from build123d import *

# Parameters (mm, degrees)
BOSS_EXTRUDE1_DEPTH       = 3
BOSS_EXTRUDE1_DEPTH_BACK  = 3
SKETCH2_R                 = 4.5
BOSS_EXTRUDE4_START       = -8.5
SKETCH2_6_R               = 6.5
SKETCH2_6_R_2             = 4.5
BOSS_EXTRUDE4_DEPTH       = 17
BOSS_EXTRUDE2_DEPTH       = 8.5
BOSS_EXTRUDE2_DEPTH_BACK  = 8.5
M2_TAPPED_HOLE1_REACH     = 63.876
M2_TAPPED_HOLE1_BORE_R    = 1.25
M2_TAPPED_HOLE2_REACH     = 59.753
M2_TAPPED_HOLE2_BORE_R    = 1.25
M3X0_5_TAPPED_HOLE1_D     = 2.5
M3X0_5_TAPPED_HOLE1_DEPTH = 7.5
M3X0_5_TAPPED_HOLE1_TIP   = 0.751075774
M3X0_5_TAPPED_HOLE2_D     = 2.5
M3X0_5_TAPPED_HOLE2_DEPTH = 7.5
M3X0_5_TAPPED_HOLE2_TIP   = 0.751075774


with BuildPart() as part:
    # Sketch2 → Boss-Extrude1 (new, two sides: drawn at the far end of the back side and taken through both)
    with BuildSketch(Plane(origin=(0, 0, 0), x_dir=(0, 0, -1), z_dir=(1, 0, 0)).offset(-BOSS_EXTRUDE1_DEPTH_BACK)):
        with BuildLine():
            ThreePointArc((0.33951151, -17.055452752), (1.492864746, -16.361954251), (1.94565571, -15.094616806))
            Line((1.94565571, -15.094616806), (1.94565571, -12.094616806))
            ThreePointArc((1.94565571, -12.094616806), (2.040471682, -11.22885835), (2.320424562, -10.404143759))
            Line((2.320424562, -10.404143759), (11.713700119, 9.73980068))
            ThreePointArc((11.713700119, 9.73980068), (12.140663851, 10.020732686), (12.599964806, 10.244927809))
            ThreePointArc((12.599964806, 10.244927809), (13.500806616, 10.98137419), (13.839273926, 12.094616806))
            Line((13.839273926, 12.094616806), (13.839273926, 15.094616806))
            ThreePointArc((13.839273926, 15.094616806), (13.500806616, 16.207859421), (12.599964806, 16.944305803))
            ThreePointArc((12.599964806, 16.944305803), (11.821767305, 17.370774506), (11.156747464, 17.958324943))
            ThreePointArc((11.156747464, 17.958324943), (9.9384514, 19.007187499), (8.5, 19.724972654))
            Line((8.5, 19.724972654), (8.5, 51.177740757))
            ThreePointArc((8.5, 51.177740757), (7.328427125, 54.006167882), (4.5, 55.177740757))
            Line((4.5, 55.177740757), (-4.5, 55.177740757))
            ThreePointArc((-4.5, 55.177740757), (-7.328427125, 54.006167882), (-8.5, 51.177740757))
            Line((-8.5, 51.177740757), (-8.5, -2.847998534))
            Line((-8.5, -2.847998534), (-12.230274542, -10.847598104))
            ThreePointArc((-12.230274542, -10.847598104), (-10.052447802, -18.929627561), (-1.717156713, -18.164740706))
            ThreePointArc((-1.717156713, -18.164740706), (-0.771632326, -17.45656389), (0.33951151, -17.055452752))
        make_face()
        with Locations((-6.339273926, -13.594616806)):
            Circle(SKETCH2_R, mode=Mode.SUBTRACT)
        with Locations((6.339273926, 13.594616806)):
            Circle(SKETCH2_R, mode=Mode.SUBTRACT)
    extrude(amount=BOSS_EXTRUDE1_DEPTH + BOSS_EXTRUDE1_DEPTH_BACK)

    # Sketch2<6> → Boss-Extrude4 (add)
    # profile 1 of 2: a face of its own
    with BuildSketch(Plane(origin=(0, 0, 0), x_dir=(0, 0, -1), z_dir=(1, 0, 0)).offset(BOSS_EXTRUDE4_START)):
        with BuildLine():
            ThreePointArc((11.156747464, 9.230908668), (11.423199363, 9.498514711), (11.713700119, 9.73980068))
            ThreePointArc((11.713700119, 9.73980068), (12.140663851, 10.020732686), (12.599964806, 10.244927809))
            ThreePointArc((12.599964806, 10.244927809), (13.500806616, 10.98137419), (13.839273926, 12.094616806))
            Line((13.839273926, 12.094616806), (13.839273926, 15.094616806))
            ThreePointArc((13.839273926, 15.094616806), (13.500806616, 16.207859421), (12.599964806, 16.944305803))
            ThreePointArc((12.599964806, 16.944305803), (11.821767305, 17.370774506), (11.156747464, 17.958324943))
            ThreePointArc((11.156747464, 17.958324943), (12.404073098, 15.933037427), (12.839273926, 13.594616806))
            ThreePointArc((12.839273926, 13.594616806), (12.404073098, 11.256196185), (11.156747464, 9.230908668))
        make_face()
    # profile 2 of 2: a face of its own
    with BuildSketch(Plane(origin=(0, 0, 0), x_dir=(0, 0, -1), z_dir=(1, 0, 0)).offset(BOSS_EXTRUDE4_START)):
        with Locations((6.339273926, 13.594616806)):
            Circle(SKETCH2_6_R)
        with Locations((6.339273926, 13.594616806)):
            Circle(SKETCH2_6_R_2, mode=Mode.SUBTRACT)
    extrude(amount=BOSS_EXTRUDE4_DEPTH)

    # Sketch2<4> → Boss-Extrude2 (add, two sides: drawn at the far end of the back side and taken through both)
    with BuildSketch(Plane(origin=(0, 0, 0), x_dir=(0, 0, -1), z_dir=(1, 0, 0)).offset(-BOSS_EXTRUDE2_DEPTH_BACK)):
        with BuildLine():
            Line((-8.5, 51.177740757), (-8.5, 30.594616806))
            ThreePointArc((-8.5, 30.594616806), (-7.328427125, 27.766189681), (-4.5, 26.594616806))
            Line((-4.5, 26.594616806), (4.5, 26.594616806))
            ThreePointArc((4.5, 26.594616806), (7.328427125, 27.766189681), (8.5, 30.594616806))
            Line((8.5, 30.594616806), (8.5, 51.177740757))
            ThreePointArc((8.5, 51.177740757), (7.328427125, 54.006167882), (4.5, 55.177740757))
            Line((4.5, 55.177740757), (-4.5, 55.177740757))
            ThreePointArc((-4.5, 55.177740757), (-7.328427125, 54.006167882), (-8.5, 51.177740757))
        make_face()
    extrude(amount=BOSS_EXTRUDE2_DEPTH + BOSS_EXTRUDE2_DEPTH_BACK)

    # M2 Tapped Hole1 bore → M2 Tapped Hole1 (cut, up to next)
    with BuildSketch(Plane(origin=(0, 0, -13.839273926), x_dir=(-1, 0, 0), z_dir=(0, 0, -1)), mode=Mode.PRIVATE) as m2_tapped_hole1_sk1:
        with Locations((0, 13.594616806)):
            Circle(M2_TAPPED_HOLE1_BORE_R)
    m2_tapped_hole1_tool1 = extrude(m2_tapped_hole1_sk1.sketch, amount=-M2_TAPPED_HOLE1_REACH, mode=Mode.PRIVATE) & part.part
    add(m2_tapped_hole1_tool1.solids().sort_by_distance((0, 13.594617, -13.839274))[0], mode=Mode.SUBTRACT)

    # M2 Tapped Hole2 bore → M2 Tapped Hole2 (cut, up to next)
    with BuildSketch(Plane(origin=(0, 0, -1.94565571), x_dir=(-1, 0, 0), z_dir=(0, 0, -1)), mode=Mode.PRIVATE) as m2_tapped_hole2_sk1:
        with Locations((0, -13.594616806)):
            Circle(M2_TAPPED_HOLE2_BORE_R)
    m2_tapped_hole2_tool1 = extrude(m2_tapped_hole2_sk1.sketch, amount=-M2_TAPPED_HOLE2_REACH, mode=Mode.PRIVATE) & part.part
    add(m2_tapped_hole2_tool1.solids().sort_by_distance((0, -13.594617, -1.945656))[0], mode=Mode.SUBTRACT)

    # M3x0.5 Tapped Hole1
    with Locations(Plane.ZY.offset(8.5)):
        with Locations((-3.5, 49.177740757), (3.5, 32.594616806)):
            Hole(M3X0_5_TAPPED_HOLE1_D / 2, depth=M3X0_5_TAPPED_HOLE1_DEPTH)
            with Locations((0, 0, -(M3X0_5_TAPPED_HOLE1_DEPTH + M3X0_5_TAPPED_HOLE1_TIP / 2))):  # 118° drill point
                Cone(0, M3X0_5_TAPPED_HOLE1_D / 2, M3X0_5_TAPPED_HOLE1_TIP, mode=Mode.SUBTRACT)

    # M3x0.5 Tapped Hole2
    with Locations(Plane(origin=(8.5, 0, 0), x_dir=(0, 0, -1), z_dir=(1, 0, 0))):
        with Locations((-3.5, 49.177740757), (3.5, 32.594616806)):
            Hole(M3X0_5_TAPPED_HOLE2_D / 2, depth=M3X0_5_TAPPED_HOLE2_DEPTH)
            with Locations((0, 0, -(M3X0_5_TAPPED_HOLE2_DEPTH + M3X0_5_TAPPED_HOLE2_TIP / 2))):  # 118° drill point
                Cone(0, M3X0_5_TAPPED_HOLE2_D / 2, M3X0_5_TAPPED_HOLE2_TIP, mode=Mode.SUBTRACT)


solid = part.part
Geometry check sheet. Reference: the model listing, model coordinates, mm. A direction names the side the tool comes from. Round coordinates to 2 decimals unless told otherwise and drop trailing zeros. Write each loop counter-clockwise with the first axis right and the second up, starting at its lowest first coordinate (ties: lowest second). Pieces come first, ordered by that corner, then holes.
Item 1: Section check B-B (z = 10). Record the boundary of the cut face in (x, y), plus the area to 3 significant figures.
Determined:
outline: (-3, -18.97) - (3, -18.97) - (3, -16.21) - (-3, -16.21) - close; (-3, -10.98) - (3, -10.98) - (3, -6.06) - (-3, -6.06) - close
area: 46.0 mm2
Item 2: Mould release check, pull along Y, two halves, no side actions. Record for faces 1 (the face through (0, 55.178, 0)), 2 (the face through (-0.042, -17.464, 0.786)), 3 (the face through (4.698, 47.957, 3.229)): +Y half, -Y half, draft (parallel to the pull), parting line (faces both ways), or undercut.
Determined:
face 1: +Y half
face 2: -Y half
face 3: undercut
Item 3: Access from +Z, -Z, +X, -X, +Y, -Y to the whole of each face (thin tool, end or side, straight path). Record for faces 4 (the face through (0, 31, 8.5)), 5 (the face through (-6, 26.595, 0)), 6 (the face through (-1.4, -13.6, -1.946)), 7 (the face through (6, 26.595, 0)), 8 (the face through (0.271, 12.374, -12.273)).
Determined:
face 4: +Z, +X, -X, +Y
face 5: +Z, -Z, -X
face 6: -Z, +X, -X, -Y
face 7: +Z, -Z, +X
face 8: -Z
Item 4: Go/stop test with flat-tipped pins: pin 1 Ø5 at (y, z) = (23.5, -2) entering from -X; pin 2 Ø5 at (x, y) = (-2.5, 42) entering from -Z; pin 3 Ø4.5 at (x, z) = (4.5, 0) entering from -Y. Record where each tip stops, or that it passes through.
Determined:
pin 1: stops at x = -3
pin 2: stops at z = -8.5
pin 3: stops at y = -18.12
Item 5: Section check A-A (x = 4). Record the boundary of the cut face in (y, z), plus the area to 3 significant figures.
Determined:
outline: (9.23, -11.16) arc R4 cw to (10.24, -12.6) arc R2 ccw to (12.09, -13.84) - (15.09, -13.84) arc R2 ccw to (16.94, -12.6) arc R4 cw to (17.96, -11.16) arc R6.5 ccw (long way) to start; (26.59, -4.5) arc R4 ccw to (30.59, -8.5) - (51.18, -8.5) arc R4 ccw to (55.18, -4.5) - (55.18, 4.5) arc R4 ccw to (51.18, 8.5) - (30.59, 8.5) arc R4 ccw to (26.59, 4.5) - close; hole circle Ø9 at (13.59, -6.34); hole circle Ø2.5 at (32.59, -3.5); hole circle Ø2.5 at (49.18, 3.5)
area: 539 mm2
Item 6: Material ranges on line 1 along Y through (x, z) = (1.75, -3.25); line 2 along Y through (x, z) = (3.75, -3.5); line 3 along X through (y, z) = (-2, 6.25), recorded low to high.
Determined:
line 1: y = -8.41 to 10.32, 16.87 to 31.37, 33.82 to 55.18
line 2: y = 7.75 to 10.1, 17.09 to 19.44, 26.59 to 31.34, 33.84 to 55.18
line 3: x = -3 to 3
Item 7: Section check C-C (y = -5). Record the boundary of the cut face in (x, z), plus the area to 3 significant figures.
Determined:
outline: (-3, -4.84) - (3, -4.84) - (3, 9.5) - (-3, 9.5) - close
area: 86.1 mm2
